Here's how the part is built. I have some questions about the finished solid (model axes, mm). Face numbers are marked on the shaded views. A direction names the side the tool comes from. Coordinates: 2 decimals unless noted, no trailing zeros. Loops run counter-clockwise (first coordinate to the right, second up) from the corner with the lowest first, then second, coordinate; pieces in that order, holes last. Notation, with made-up numbers: M 5,16 L 57,16 A26 cw 57,32 Z; hole C 49,56 d11. An arc over 180 degrees is marked long. Use CSV: the item, a comma, the result in double quotes. Start each with the question number.
Q1. If we section it at A-A (x = 5.5): Please give me the cut outline in (y, z), and give its area (3 significant figures).
Q2. If we section it at B-B (y = -2.25): Please give me the cut outline in (x, z).
Q3. If we section it at C-C (z = 27): Please give me the cut outline in (x, y), and give its area (3 significant figures).
Q4. If we mould it in two halves opening along Y, with no side actions, what happens to the marked faces 1, 2 and 3? For each: +Y half, -Y half, draft (parallel to the pull), parting line (faces both ways), or undercut.
Q5. If we section it at D-D (y = 3.5): Please give me the cut outline in (x, z), and give its area (3 significant figures).
Q6. For pin 1 Ø8 at (x, y) = (-6, 5) entering from -Z; pin 2 Ø5 at (x, z) = (-8.5, -3.5) entering from -Y; pin 3 Ø2 at (y, z) = (-0.5, -5.5) entering from -X, each with a flat end and sliding along its axis, tell me the tip position at first contact or that it passes through.
Q7. Please list where these lines run through material, in increasing order: probe 1 along Y at (x, z) = (11, 24); probe 2 along X at (y, z) = (7.75, 32); probe 3 along Z at (x, y) = (6.75, -1). Write a range as [from, to].
Q8. Which directions (+Z, -Z, +X, -X, +Y, -Y) give clear straight access to the entire face, cutting with the end or side of a thin tool? Please do the marked faces 4, 5 and 6.
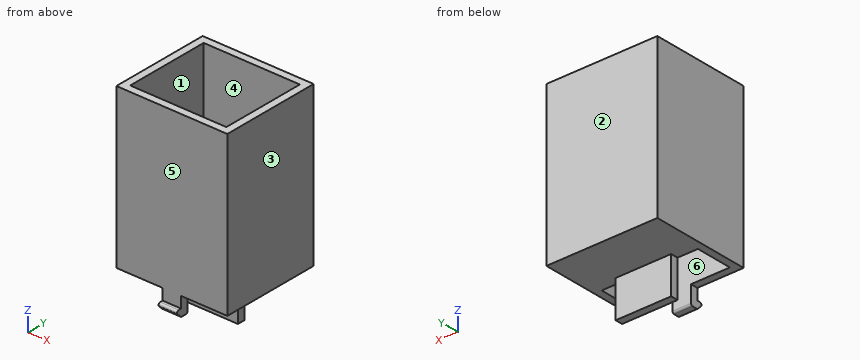
from build123d import *

# Parameters (mm, degrees)
SKETCH1_W           = 30
SKETCH1_H           = 27
SKETCH1_W_2         = 26
SKETCH1_H_2         = 23
BOSS_EXTRUDE1_DEPTH = 43
SKETCH3_W           = 30
SKETCH3_H           = 15
BOSS_EXTRUDE2_DEPTH = 2
SKETCH5_W           = 15
SKETCH5_H           = 2
SKETCH5_W_2         = 5
BOSS_EXTRUDE3_DEPTH = 10
BOSS_EXTRUDE4_DEPTH = 5
SKETCH7_W           = 5
SKETCH7_H           = 2
CUT_EXTRUDE1_DEPTH  = 5
FILLET3_R           = 0.5


with BuildPart() as part:
    # Sketch1 → Boss-Extrude1 (new body)
    with BuildSketch(Plane.XY):
        Rectangle(SKETCH1_W, SKETCH1_H)
        Rectangle(SKETCH1_W_2, SKETCH1_H_2, mode=Mode.SUBTRACT)
    extrude(amount=BOSS_EXTRUDE1_DEPTH)

    # Sketch3 → Boss-Extrude2 (add)
    with BuildSketch(Plane(origin=(0, 0, 0), x_dir=(-1, 0, 0), z_dir=(0, 0, -1))):
        with Locations((0, 6)):
            Rectangle(SKETCH3_W, SKETCH3_H)
    extrude(amount=-BOSS_EXTRUDE2_DEPTH)

    # Sketch5 → Boss-Extrude3 (add)
    with BuildSketch(Plane(origin=(0, 0, 0), x_dir=(-1, 0, 0), z_dir=(0, 0, -1))):
        with Locations((0, -0.5)):
            Rectangle(SKETCH5_W, SKETCH5_H)
        with Locations((0, -12.5)):
            Rectangle(SKETCH5_W_2, SKETCH5_H)
    extrude(amount=BOSS_EXTRUDE3_DEPTH)

    # Sketch6 → Boss-Extrude4 (add)
    with BuildSketch(Plane.ZY.offset(2.5)):
        Polygon((-5, -13.5), (-3, -15.5), (-3, -13.5), align=None)
    extrude(amount=-BOSS_EXTRUDE4_DEPTH)

    # Sketch7 → Cut-Extrude1 (cut)
    with BuildSketch(Plane(origin=(0, 0, -10), x_dir=(-1, 0, 0), z_dir=(0, 0, -1))):
        with Locations((0, -12.5)):
            Rectangle(SKETCH7_W, SKETCH7_H)
    extrude(amount=-CUT_EXTRUDE1_DEPTH, mode=Mode.SUBTRACT)

    # Fillet3
    fillet3_edges = [part.edges().sort_by_distance(p)[0] for p in [
        (0, -13.5, -5),
        (0, -15.5, -3),
        (0, -11.5, -5),
    ]]
    fillet(fillet3_edges, radius=FILLET3_R)


solid = part.part
Results below:
1,outline,"M -13.5,0 L -11.5,0 L -11.5,43 L -13.5,43 Z; M -1.5,-10 L 0.5,-10 L 0.5,0 L 13.5,0 L 13.5,43 L 11.5,43 L 11.5,2 L -1.5,2 Z"
1,area,"218 mm^2"
2,outline,"M -15,0 L -13,0 L -13,43 L -15,43 Z; M 13,0 L 15,0 L 15,43 L 13,43 Z"
3,outline,"M -15,-13.5 L 15,-13.5 L 15,13.5 L -15,13.5 Z; hole M -13,-11.5 L 13,-11.5 L 13,11.5 L -13,11.5 Z"
3,area,"212 mm^2"
4,face 1,"undercut"
4,face 2,"+Y half"
4,face 3,"draft"
5,outline,"M -15,0 L 15,0 L 15,43 L 13,43 L 13,2 L -13,2 L -13,43 L -15,43 Z"
5,area,"224 mm^2"
6,pin 1,"z = 0"
6,pin 2,"y = -1.5"
6,pin 3,"x = -7.5"
7,probe 1,"[-13.5, -11.5], [11.5, 13.5]"
7,probe 2,"[-15, -13], [13, 15]"
7,probe 3,"[-10, 2]"
8,face 4,"+Z"
8,face 5,"+Z, +X, -X, -Y"
8,face 6,"+Z, -Z"
